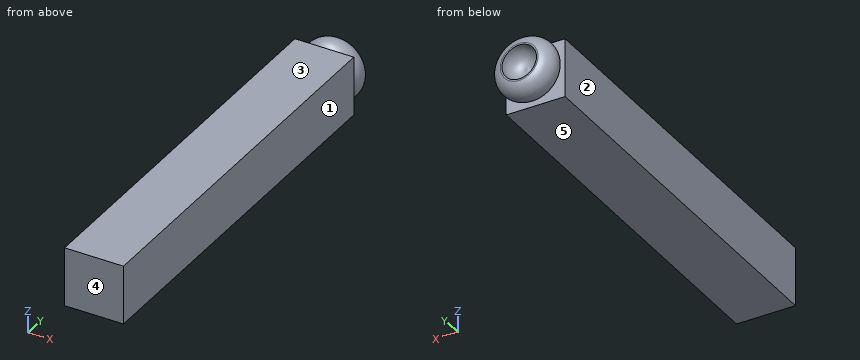
```python
from build123d import *

# Parameters (mm, degrees)
SKETCH4_W           = 19.05
SKETCH4_H           = 19.05
BOSS_EXTRUDE1_DEPTH = 127


with BuildPart() as part:
    # Sketch2 → Revolve2 (revolve)
    with BuildSketch(Plane.XY, mode=Mode.PRIVATE) as revolve2_sk:
        with BuildLine():
            Line((0, 8.168367528), (0, 3.636735056))
            Line((0, 3.636735056), (4.947214611, 3.636735056))
            ThreePointArc((4.947214611, 3.636735056), (9.865040683, 7.617829413), (6.096, 12.7))
            Line((6.096, 12.7), (5.588, 12.7))
            ThreePointArc((5.588, 12.7), (3.946698626, 9.012779896), (0, 8.168367528))
        make_face()
    revolve(revolve2_sk.sketch.rotate(Axis((0, 3.636735056, 0), (0, 1, 0)), 90), axis=Axis((0, 3.636735056, 0), (0, 1, 0)))

    # Sketch4 → Boss-Extrude1 (add)
    with BuildSketch(Plane.XZ.offset(-3.636735056)):
        Rectangle(SKETCH4_W, SKETCH4_H)
    extrude(amount=BOSS_EXTRUDE1_DEPTH)


solid = part.part
```
Geometry: final body of the model. Coordinates: model frame, mm. Face numbers are marked on the shaded views. A direction names the side the tool comes from. Round coordinates to 2 decimals unless told otherwise and drop trailing zeros. Write each loop counter-clockwise with the first axis right and the second up, starting at its lowest first coordinate (ties: lowest second). Pieces come first, ordered by that corner, then holes. Notation, with made-up numbers: (-34, 13) -> (21, 13) arc R21 cw to (21, 41) -> close; hole circle Ø1 at (-34, 5). An arc over 180 degrees is marked (long way). Return JSON: item names as keys, results as strings.
Q1. Section A-A on y = -53.5. Return the cut outline in (x, z) (3 decimals).
From the geometry:
{"outline": "(-9.525, -9.525) -> (9.525, -9.525) -> (9.525, 9.525) -> (-9.525, 9.525) -> close"}
Q2. Ray query, line 1 (X direction, y = -70, z = -8.25) (3 decimals); line 2 (Y direction, x = 5.5, z = -6). Return the intervals inside material, ascending.
From the geometry:
{"line 1": "-9.525 to 9.525", "line 2": "-123.36 to 3.64, 4.59 to 11.8"}
Q3. Set-up query: the marked faces 1, 2, 3, 4 and 5. Return all of +Z, -Z, +X, -X, +Y, -Y with unobstructed straight access to the full face (end or side cutting, diameter ignored); none if empty.
From the geometry:
{"face 1": "+Z, -Z, +X, -Y", "face 2": "+Z, -Z, -X, -Y", "face 3": "+Z, +X, -X, -Y", "face 4": "+Z, -Z, +X, -X, -Y", "face 5": "-Z, +X, -X, -Y"}
Q4. First-contact query: pin 1 Ø5.5 at (y, z) = (-81, -2.5) entering from +X (3 decimals); pin 2 Ø1 at (x, y) = (-2, -11.5) entering from -Z (3 decimals); pin 3 Ø5.5 at (y, z) = (-50, 1) entering from -X (3 decimals); pin 4 Ø5.5 at (x, z) = (4.5, 0) entering from +Y. Flat tips, straight axial feed; report the tip coordinate or a pass-through.
From the geometry:
{"pin 1": "x = 9.525", "pin 2": "z = -9.525", "pin 3": "x = -9.525", "pin 4": "y = 12.7"}
